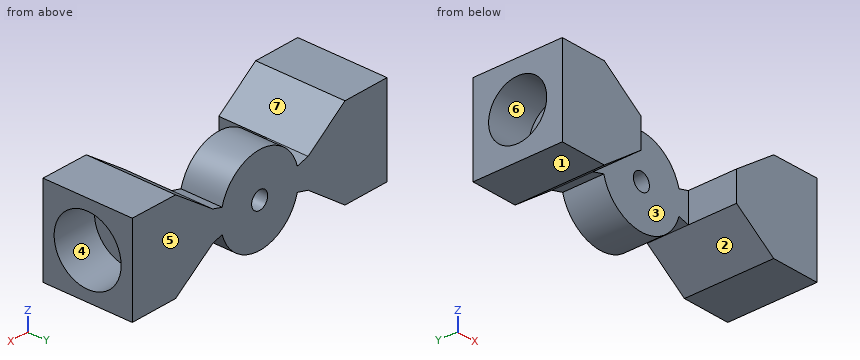
```python
from build123d import *

# Parameters (mm, degrees)
F1_DEPTH = 12.7
F3_DEPTH = 6.858
F4_R     = 4.130232
F5_DEPTH = 6.35
F6_R     = 4.764812
F7_DEPTH = 6.35
F8_R     = 1.264883
F9_DEPTH = 25.4


with BuildPart() as f1:
    # F0 (on Front) → F1 (new body)
    with BuildSketch(Plane.XZ):
        Polygon((-7.644902, -2.058817), (-7.644902, 2.058817), (-13.462164, 6.35), (-20.092922, 6.35), (-20.092922, 0), (-20.092922, -6.35), (-13.462164, -6.35), align=None)
        with BuildLine():
            Line((7.394814, 2.058817), (5.928265, 1.65051))
            ThreePointArc((5.928265, 1.65051), (-0.026068, 6.153685), (-5.942036, 1.600225))
            Line((-5.942036, 1.600225), (-7.644902, 2.058817))
            Line((-7.644902, 2.058817), (-7.644902, -2.058817))
            Line((-7.644902, -2.058817), (-5.942036, -1.600225))
            ThreePointArc((-5.942036, -1.600225), (-0.051739, -6.153522), (5.914289, -1.699913))
            Line((5.914289, -1.699913), (7.394814, -2.125453))
            Line((7.394814, -2.125453), (7.394814, 2.058817))
        make_face()
        Polygon((13.260647, 6.283364), (7.394814, 2.058817), (7.394814, -2.125453), (13.260647, -6.35), (20.092922, -6.35), (20.092922, 0), (20.092922, 6.35), align=None)
    extrude(amount=F1_DEPTH)

    # F2 (on face) → F3 (cut)
    with BuildSketch(Plane.XZ.offset(12.7)):
        with BuildLine():
            Line((-5.942036, 1.600225), (-7.644902, 2.058817))
            Line((-7.644902, 2.058817), (-7.644902, -2.058817))
            Line((-7.644902, -2.058817), (-5.942036, -1.600225))
            ThreePointArc((-5.942036, -1.600225), (-0.051739, -6.153522), (5.914289, -1.699913))
            Line((5.914289, -1.699913), (7.394814, -2.125453))
            Line((7.394814, -2.125453), (7.394814, 2.058817))
            Line((7.394814, 2.058817), (5.928265, 1.65051))
            ThreePointArc((5.928265, 1.65051), (-0.026068, 6.153685), (-5.942036, 1.600225))
        make_face()
    extrude(amount=-F3_DEPTH, mode=Mode.SUBTRACT)

    # F4 (on face) → F5 (cut)
    with BuildSketch(Plane(origin=(-20.092922, 0, 0), x_dir=(0, -1, 0), z_dir=(-1, 0, 0))):
        with Locations((6.35, 0)):
            Circle(F4_R)
    extrude(amount=-F5_DEPTH, mode=Mode.SUBTRACT)

    # F6 (on face) → F7 (cut)
    with BuildSketch(Plane.YZ.offset(20.092922)):
        with Locations((-6.349694, 0)):
            Circle(F6_R)
    extrude(amount=-F7_DEPTH, mode=Mode.SUBTRACT)

    # F8 (on face) → F9 (cut)
    with BuildSketch(Plane.XZ.offset(5.842)):
        Circle(F8_R)
    extrude(amount=-F9_DEPTH, mode=Mode.SUBTRACT)


solid = f1.part
```
Work out the finished part from the listing and answer in its coordinate system (mm). Face numbers are marked on the shaded views. A direction names the side the tool comes from. Round coordinates to 2 decimals unless told otherwise and drop trailing zeros. Order: outer loops, then holes, each group sorted by start corner. A loop starts at its lowest first (then second) coordinate and runs counter-clockwise, first axis right, second up.
Q1. A cutting plane is placed at B-B, the plane x = 0. Determine the outline of the cut face in (y, z).
Solution:
outline: (-5.84, -6.15) - (0, -6.15) - (0, -1.26) - (-5.84, -1.26) - close; (-5.84, 1.26) - (0, 1.26) - (0, 6.15) - (-5.84, 6.15) - close
Q2. Given pin 1 Ø3.5 at (x, z) = (-1, -0.5) entering from -Y; pin 2 Ø3 at (x, y) = (0, -4) entering from +Z; pin 3 Ø3.5 at (y, z) = (-8.5, 0) entering from -X, each flat-ended and moving along its own axis, determine where each tip first touches the part or whether it passes through.
Solution:
pin 1: stops at y = -5.84
pin 2: stops at z = 6.15
pin 3: stops at x = -13.74
Q3. The mould has two halves that part along Y. Classify the marked faces 4, 5, 6 and 7: pulls with the +Y half, pulls with the -Y half, needs draft (parallel to the pull), parting line crosses it, or undercut.
Solution:
face 4: undercut
face 5: pulls with the +Y half
face 6: undercut
face 7: needs draft
Q4. A cutting plane is placed at C-C, the plane y = -6.35. Determine the outline of the cut face in (x, z), then the cut area to 3 significant figures.
Solution:
outline: (-20.09, -6.35) - (-13.46, -6.35) - (-7.64, -2.06) - (-7.64, 2.06) - (-13.46, 6.35) - (-20.09, 6.35) - (-20.09, 4.13) - (-13.74, 4.13) - (-13.74, -4.13) - (-20.09, -4.13) - close; (7.39, -2.13) - (13.26, -6.35) - (20.09, -6.35) - (20.09, -4.76) - (13.74, -4.76) - (13.74, 4.76) - (20.09, 4.76) - (20.09, 6.35) - (13.26, 6.28) - (7.39, 2.06) - close
area: 156 mm2
Q5. A cutting plane is placed at D-D, the plane y = -1. Determine the outline of the cut face in (x, z), then the cut area to 3 significant figures.
Solution:
outline: (-20.09, -6.35) - (-13.46, -6.35) - (-7.64, -2.06) - (-5.94, -1.6) arc R6.15 ccw to (5.91, -1.7) - (7.39, -2.13) - (13.26, -6.35) - (20.09, -6.35) - (20.09, 6.35) - (13.26, 6.28) - (7.39, 2.06) - (5.93, 1.65) arc R6.15 ccw to (-5.94, 1.6) - (-7.64, 2.06) - (-13.46, 6.35) - (-20.09, 6.35) - close; hole circle Ø2.53 at (0, 0)
area: 394 mm2
Q6. Find the intervals of material crossed by line 1 along Z through (x, y) = (0, -4.4); line 2 along X through (y, z) = (-1.25, 2.5); line 3 along X through (y, z) = (-2.5, -4.75), in increasing order.
Solution:
line 1: z = -6.15 to -1.26, 1.26 to 6.15
line 2: x = -20.09 to -8.24, -5.62 to 5.62, 8.01 to 20.09
line 3: x = -20.09 to -11.29, -3.91 to 3.91, 11.04 to 20.09
Q7. A tool of negligible diameter and unlimited length cuts with its end or side. For the marked faces 1, 2 and 3, from which of +Z, -Z, +X, -X, +Y, -Y can it reach the whole face along a straight path? Write none if from no direction.
Solution:
face 1: -Z, +X, -X, +Y, -Y
face 2: -Z, +Y, -Y
face 3: +Z, -Z, -Y
Q8. A cutting plane is placed at A-A, the plane z = 0. Determine the outline of the cut face in (x, y).
Solution:
outline: (-20.09, -12.7) - (-7.64, -12.7) - (-7.64, -5.84) - (-1.26, -5.84) - (-1.26, 0) - (-20.09, 0) - (-20.09, -2.22) - (-13.74, -2.22) - (-13.74, -10.48) - (-20.09, -10.48) - close; (1.26, -5.84) - (7.39, -5.84) - (7.39, -12.7) - (20.09, -12.7) - (20.09, -11.11) - (13.74, -11.11) - (13.74, -1.58) - (20.09, -1.58) - (20.09, 0) - (1.26, 0) - close
